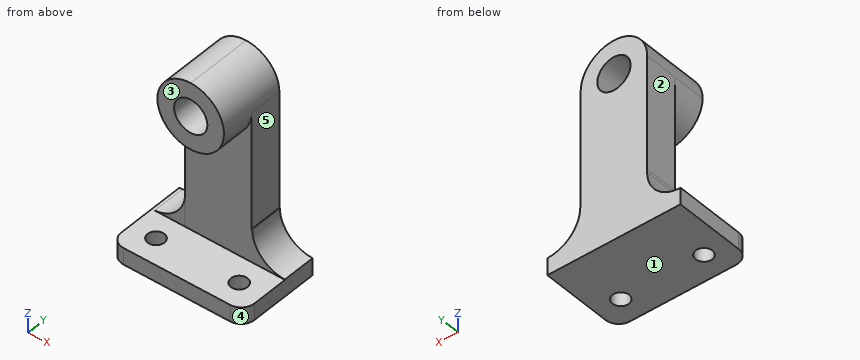
from build123d import *

# Parameters (mm, degrees)
F0_W      = 50.8
F0_H      = 31.75
F1_DEPTH  = 6.35
F2_R      = 3.175
F3_DEPTH  = 25.4
F4_R      = 5.08
F5_W      = 25.4
F5_H      = 12.7
F6_DEPTH  = 69.85
F7_R      = 6.35
F8_DEPTH  = 12.7
F9_DEPTH  = 25.4
F10_W     = 12.7
F10_H     = 12.7
F11_DEPTH = 12.7
F13_DEPTH = 25.4
F14_W     = 12.7
F14_H     = 12.7
F15_DEPTH = 12.7
F17_DEPTH = 25.4


with BuildPart() as f1:
    # F0 (on Top) → F1 (new body)
    with BuildSketch(Plane.XY):
        with Locations((-4.5064515435, 15.875)):
            Rectangle(F0_W, F0_H)
    extrude(amount=F1_DEPTH)

    # F2 (on face) → F3 (cut)
    with BuildSketch(Plane.XY.offset(6.35)):
        with Locations((11.3685484565, 9.525)):
            Circle(F2_R)
        with Locations((-20.3814515435, 9.525)):
            Circle(F2_R)
    extrude(amount=-F3_DEPTH, mode=Mode.SUBTRACT)

    # F4
    f4_edges = [f1.edges().sort_by_distance(p)[0] for p in [
        (20.893548, 0, 3.175),
        (-29.906452, 0, 3.175),
    ]]
    fillet(f4_edges, radius=F4_R)

    # F5 (on face) → F6 (join)
    with BuildSketch(Plane.XY.offset(6.35)):
        with Locations((-4.5064515435, 25.4)):
            Rectangle(F5_W, F5_H)
    extrude(amount=F6_DEPTH)

    # F7 (on face) → F8 (join)
    with BuildSketch(Plane.XZ.offset(-19.05)):
        with BuildLine():
            ThreePointArc((-17.2064515435, 63.5), (-4.5064515435, 50.8), (8.1935484565, 63.5))
            ThreePointArc((8.1935484565, 63.5), (4.473804616, 72.4802560826), (-4.5064514347, 76.2))
            ThreePointArc((-4.5064514347, 76.2), (-13.4867076261, 72.4802561595), (-17.2064515435, 63.5))
        make_face()
        with Locations((-4.5064515435, 63.5)):
            Circle(F7_R, mode=Mode.SUBTRACT)
    extrude(amount=F8_DEPTH)

    # F9 (cut): faces of the model
    f9_faces = [f1.faces().sort_by_distance(p)[0] for p in [
        (5.3567756319, 19.05, 73.3632271754),
        (-14.3696787189, 19.05, 73.3632271754),
        (-4.5064515435, 19.05, 63.5),
    ]]
    extrude(f9_faces, amount=-F9_DEPTH, mode=Mode.SUBTRACT)

    # F10 (on face) → F11 (join)
    with BuildSketch(Plane.YZ.offset(8.1935484565)):
        with Locations((25.4, 12.7)):
            Rectangle(F10_W, F10_H)
    extrude(amount=F11_DEPTH)

    # F12 (on face) → F13 (cut)
    with BuildSketch(Plane.XZ.offset(-19.05)):
        with BuildLine():
            ThreePointArc((33.4102507488, 19.05), (20.8935484565, 31.5667022923), (8.3768461642, 19.05))
            Line((8.3768461642, 19.05), (20.8935484565, 19.05))
            Line((20.8935484565, 19.05), (20.8935484565, 6.5332977077))
            ThreePointArc((20.8935484565, 6.5332977077), (29.7441935255, 10.199354931), (33.4102507488, 19.05))
        make_face()
        with BuildLine():
            Line((20.8935484565, 19.05), (8.3768461642, 19.05))
            ThreePointArc((8.3768461642, 19.05), (12.0429033875, 10.199354931), (20.8935484565, 6.5332977077))
            Line((20.8935484565, 6.5332977077), (20.8935484565, 19.05))
        make_face()
    extrude(amount=-F13_DEPTH, mode=Mode.SUBTRACT)

    # F14 (on face) → F15 (join)
    with BuildSketch(Plane(origin=(-17.2064515435, 0, 0), x_dir=(0, -1, 0), z_dir=(-1, 0, 0))):
        with Locations((-25.4, 12.7)):
            Rectangle(F14_W, F14_H)
    extrude(amount=F15_DEPTH)

    # F16 (on face) → F17 (cut)
    with BuildSketch(Plane.XZ.offset(-19.05)):
        with BuildLine():
            ThreePointArc((-28.8202851524, 6.35), (-20.5172442286, 10.4295276564), (-17.1600890259, 19.05))
            ThreePointArc((-17.1600890259, 19.05), (-17.17168493, 19.5935777111), (-17.2064515435, 20.1361663911))
            Line((-17.2064515435, 20.1361663911), (-17.2064515435, 19.05))
            Line((-17.2064515435, 19.05), (-29.9064515435, 19.05))
            Line((-29.9064515435, 19.05), (-29.9064515435, 6.35))
            Line((-29.9064515435, 6.35), (-28.8202851524, 6.35))
        make_face()
    extrude(amount=-F17_DEPTH, mode=Mode.SUBTRACT)


solid = f1.part
Can you work these out from the model? Positions are in its coordinate system, mm. Face numbers are marked on the shaded views. A direction names the side the tool comes from. Round coordinates to 2 decimals unless told otherwise and drop trailing zeros. Write each loop counter-clockwise with the first axis right and the second up, starting at its lowest first coordinate (ties: lowest second). Pieces come first, ordered by that corner, then holes. Notation, with made-up numbers: (57.25, 0.25) - (61.25, 0.25) arc R22 ccw to (61.25, 9.25) - close; hole circle Ø3 at (-27.5, 87.25). An arc over 180 degrees is marked (long way). Write each question's results on one line, items separated by ' | '. Start each with the question number.
1) For pin 1 Ø5 at (y, z) = (12.5, 60.5) entering from -X; pin 2 Ø12 at (x, y) = (11.5, 4) entering from +Z; pin 3 Ø10 at (y, z) = (17, 40) entering from +X, each with a flat end and sliding along its axis, tell me the tip position at first contact or that it passes through.
2) Suppose I cut it at B-B (y = 22). List the corners of the cut face in (x, z) for me.
3) Suppose I cut it at D-D (y = 7.5). List the corners of the cut face in (x, z) for me.
4) Which directions (+Z, -Z, +X, -X, +Y, -Y) give clear straight access to the entire face, cutting with the end or side of a thin tool? Please do the marked faces 1, 2, 3, 4 and 5.
5) Suppose I cut it at A-A (y = 14). List the corners of the cut face in (x, z) for me.
6) Please list where these lines run through material, in increasing order: line 1 (X direction, y = 11, z = 63); line 2 (X direction, y = 28, z = 66); line 3 (Y direction, x = 4, z = 39).
7) Suppose I cut it at C-C (x = -10). List the corners of the cut face in (y, z) for me, and give its area (3 significant figures).
Here are the results:
1) pin 1: stops at x = -17.2 | pin 2: stops at z = 70.67 | pin 3: stops at x = 8.19
2) outline: (-29.91, 0) - (20.89, 0) - (20.89, 6.53) arc R12.52 cw to (8.38, 19.05) - (8.19, 19.05) - (8.19, 63.5) arc R12.7 ccw to (-17.21, 63.5) - (-17.21, 20.14) arc R12.75 cw to (-28.82, 6.35) - (-29.91, 6.35) - close; hole circle Ø12.7 at (-4.51, 63.5)
3) outline: (-29.91, 0) - (-22.83, 0) - (-22.83, 6.35) - (-29.91, 6.35) - close; (-17.94, 0) - (8.92, 0) - (8.92, 6.35) - (-17.94, 6.35) - close; circle Ø25.4 at (-4.51, 63.5); (13.81, 0) - (20.89, 0) - (20.89, 6.35) - (13.81, 6.35) - close; hole circle Ø12.7 at (-4.51, 63.5)
4) face 1: -Z, +X, -X, +Y, -Y | face 2: +Z, -X, +Y, -Y | face 3: +Z, +X, -X, -Y | face 4: +Z, -Z, +X, -Y | face 5: +Z, +X, +Y, -Y
5) outline: (-29.91, 0) - (20.89, 0) - (20.89, 6.35) - (-29.91, 6.35) - close; circle Ø25.4 at (-4.51, 63.5); hole circle Ø12.7 at (-4.51, 63.5)
6) line 1: x = -17.2 to -10.84, 1.82 to 8.18 | line 2: x = -16.96 to -10.34, 1.33 to 7.95 | line 3: y = 19.05 to 31.75
7) outline: (0, 0) - (31.75, 0) - (31.75, 60.32) - (6.35, 60.32) - (6.35, 52.05) - (19.05, 52.05) - (19.05, 6.35) - (0, 6.35) - close; (6.35, 66.68) - (31.75, 66.68) - (31.75, 74.95) - (6.35, 74.95) - close | area: 1,200 mm2
